```python
from build123d import *

# Parameters (mm, degrees)
F0_W     = 20
F0_H     = 28.5
F1_DEPTH = 4
F3_START = 12.6
F2_R     = 2.4616630518
F3_DEPTH = 6.8


with BuildPart() as f1:
    # F0 (on Top) → F1 (new body)
    with BuildSketch(Plane.XY):
        Rectangle(F0_W, F0_H)
    extrude(amount=F1_DEPTH)

    # F2 (on Front) → F3 (join)
    with BuildSketch(Plane.XZ.offset(F3_START)):
        with Locations((0, 1.8549020169)):
            Circle(F2_R)
    extrude(amount=F3_DEPTH)


solid = f1.part
```
Can you work these out from the model? Positions are in its coordinate system, mm. A direction names the side the tool comes from. Coordinates: 2 decimals unless noted, no trailing zeros. Loops run counter-clockwise (first coordinate to the right, second up) from the corner with the lowest first, then second, coordinate; pieces in that order, holes last. Notation, with made-up numbers: M 36,-29.75 L 71,-29.75 A9 ccw 71,-24.75 Z; hole C -3,66 d3. An arc over 180 degrees is marked long. Put each result on its own line as item: value. Start each with the question number.
(1) Will these pins go through, and if not, where does the flat tip stop? pin 1 Ø0.5 at (x, z) = (0.5, -0.5) entering from +Y; pin 2 Ø10 at (x, y) = (3.5, 5) entering from -Z; pin 3 Ø2 at (x, z) = (7.5, 1.5) entering from -Y.
(2) Which directions (+Z, -Z, +X, -X, +Y, -Y) give clear straight access to the entire face, cutting with the end or side of a thin tool? Please do faces 1 (the face through (-10, 0, 2)), 2 (the face through (-0.53, -16.71, -0.55)).
(3) Imagine slicing it at B-B on z = 0.6. List the corners of the cut face in (x, y) for me.
(4) Imagine slicing it at C-C on y = -11.5. List the corners of the cut face in (x, z) for me, and give its area (3 significant figures).
(5) I need wall thicknesses on probe 1 along Y at (x, z) = (5, 1.9); probe 2 along Z at (x, y) = (2.5, -11.5); probe 3 along X at (y, z) = (-17, 2.7). Which ranges of each line are inside material? Lowest first, please.
(6) Imagine slicing it at A-A on x = 0. List the corners of the cut face in (y, z) for me.
(7) Imagine slicing it at D-D on x = 4.5. List the corners of the cut face in (y, z) for me.
Worked answers:
1. pin 1: stops at y = -12.6
1. pin 2: stops at z = 0
1. pin 3: stops at y = -14.25
2. face 1: +Z, -Z, -X, +Y, -Y
2. face 2: -Y
3. outline: M -10,-14.25 L -2.12,-14.25 L -2.12,-19.4 L 2.12,-19.4 L 2.12,-14.25 L 10,-14.25 L 10,14.25 L -10,14.25 Z
4. outline: M -10,0 L 10,0 L 10,4 L -10,4 Z
4. area: 80.0 mm2
5. probe 1: y = -14.25 to 14.25
5. probe 2: z = 0 to 4
5. probe 3: x = -2.31 to 2.31
6. outline: M -19.4,-0.61 L -12.6,-0.61 L -12.6,0 L 14.25,0 L 14.25,4 L -12.6,4 L -12.6,4.32 L -19.4,4.32 Z
7. outline: M -14.25,0 L 14.25,0 L 14.25,4 L -14.25,4 Z
